Here's how the part is built. I have some questions about the finished solid (model axes, mm). A direction names the side the tool comes from. Give positions to 0.01 mm unless a question says otherwise; leave off trailing zeros. Write each loop counter-clockwise with the first axis right and the second up, starting at its lowest first coordinate (ties: lowest second). Pieces come first, ordered by that corner, then holes. Notation, with made-up numbers: (25.25, 17) - (56.25, 17) arc R14 cw to (56.25, 28) - close; hole circle Ø2 at (-13.75, 16.5). An arc over 180 degrees is marked (long way). Write each question's results on one line, items separated by ' | '. Start each with the question number.
Item 1: Suppose I cut it at B-B on y = -65.5. List the corners of the cut face in (x, z) for me.
Item 2: Will this pin go through, and if not, where does the flat tip stop? P1, Ø6, axis at x = 89, y = -213.5, coming from the -Z side.
Item 3: Suppose I cut it at D-D on y = -194.5. List the corners of the cut face in (x, z) for me.
Item 4: We'd pull the mould along X, two halves only. Please class faces 4 (the flat face through (17, -123, 0)), 5 (the flat face through (22.81, -219.12, 9.86)), 6 (the flat face through (150, -127, 17)): +X half, -X half, draft (parallel to the pull), parting line (faces both ways), or undercut.
Item 5: Suppose I cut it at A-A on x = 75. List the corners of the cut face in (y, z) for me.
Item 6: Please list where these lines run through material, in increasing order: line 1 along Y through (x, z) = (75, 27); line 2 along Z through (x, y) = (124.5, -227); line 3 along X through (y, z) = (-54, 8).
Item 7: Suppose I cut it at C-C on x = 59. List the corners of the cut face in (y, z) for me, then the cut area to 3 significant figures.
Item 8: Which directions (+Z, -Z, +X, -X, +Y, -Y) give clear straight access to the entire face, cutting with the end or side of a thin tool? Please do faces 1 (the flat face through (22.182, -67.139, 9.86)), 2 (the flat face through (127.818, -219.97, 9.86)), 3 (the flat face through (74, -123, 20)).
```python
from build123d import *

# Parameters (mm, degrees)
SKETCH_1_W          = 150
SKETCH_1_H          = 250
EXTRUDE_1_DEPTH     = 35
CUT_EXTRUDE_1_DEPTH = 20
SKETCH_3_R          = 2.5
CUT_EXTRUDE_2_DEPTH = 293.232783924


with BuildPart() as part:
    # Эскиз1 → Бобышка-Вытянуть1 (new body)
    with BuildSketch(Plane.XY):
        with Locations((75, -125)):
            Rectangle(SKETCH_1_W, SKETCH_1_H)
    extrude(amount=EXTRUDE_1_DEPTH)

    # Эскиз2 → Вырез-Вытянуть1 (cut)
    with BuildSketch(Plane.XY):
        with BuildLine():
            Line((0, 0), (44.994645372, -136.185163226))
            ThreePointArc((44.994645372, -136.185163226), (35, -162.636603521), (44.994645372, -189.088043815))
            Line((44.994645372, -189.088043815), (0, -250))
            Line((0, -250), (150, -250))
            Line((150, -250), (105.005354628, -189.088043815))
            ThreePointArc((105.005354628, -189.088043815), (115, -162.636603521), (105.005354628, -136.185163226))
            Line((105.005354628, -136.185163226), (150, 0))
            Line((150, 0), (0, 0))
        make_face()
    extrude(amount=CUT_EXTRUDE_1_DEPTH, mode=Mode.SUBTRACT)

    # Эскиз3 → Вырез-Вытянуть2 (cut, through all)
    with BuildSketch(Plane(origin=(0, 0, 20), x_dir=(-1, 0, 0), z_dir=(0, 0, -1))):
        with Locations((-75, -162.636603521)):
            Circle(SKETCH_3_R)
    extrude(amount=-CUT_EXTRUDE_2_DEPTH, mode=Mode.SUBTRACT)


solid = part.part
```
Checked values:
1) outline: (0, 0) - (21.64, 0) - (21.64, 20) - (128.36, 20) - (128.36, 0) - (150, 0) - (150, 35) - (0, 35) - close
2) P1: stops at z = 20
3) outline: (0, 0) - (41, 0) - (41, 20) - (109, 20) - (109, 0) - (150, 0) - (150, 35) - (0, 35) - close
4) face 4: draft | face 5: undercut | face 6: +X half
5) outline: (-250, 20) - (-165.14, 20) - (-165.14, 35) - (-250, 35) - close; (-160.14, 20) - (0, 20) - (0, 35) - (-160.14, 35) - close
6) line 1: y = -250 to -165.14, -160.14 to 0 | line 2: z = 20 to 35 | line 3: x = 0 to 17.84, 132.16 to 150
7) outline: (-250, 20) - (0, 20) - (0, 35) - (-250, 35) - close | area: 3,750 mm^2
8) face 1: -Z, +Y | face 2: -Z, -Y | face 3: -Z
